Could you check a few things on this drawing? It's one solid part, dimensions in mm from its lowest x, y, z. A direction names the side the tool comes from. Give positions to 0.01 mm unless a question says otherwise; leave off trailing zeros. Write each loop counter-clockwise with the first axis right and the second up, starting at its lowest first coordinate (ties: lowest second). Pieces come first, ordered by that corner, then holes.
1. Suppose I cut it at C-C (x = 24.6). Please give me the cut outline in (y, z), and give its area (3 significant figures).
2. Suppose I cut it at B-B (z = 18). Please give me the cut outline in (x, y), and give its area (4 significant figures).
3. On a 3-axis mill with a long thin cutter (end or side, diameter ignored), from which of +Z, -Z, +X, -X, +Y, -Y can I reach the whole of each face in a straight line? I mean the marked faces 1, 2 and 3. Say none if no direction works.
4. Thinking about a two-plate mould opening in Z: for the marked faces 4, 5 and 6, which applies, pulls with the +Z half, pulls with the -Z half, needs draft (parallel to the pull), parting line crosses it, or undercut?
5. Suppose I cut it at D-D (x = 7). Please give me the cut outline in (y, z), and give its area (3 significant figures).
6. I'm going to push flat-ended pins straight in: pin 1 (0.9 mm diameter, centred on y = 19, z = 1.5, fed in from +X); pin 2 (0.9 mm diameter, centred on y = 17, z = 22.5, fed in from -X); pin 3 (3 mm diameter, centred on x = 23, z = 15.5, fed in from -Y). Where does each tip first touch, or does it pass through?
7. If I drill on probe 1 along Y at (x, z) = (10.8, 21.9); probe 2 along Z at (x, y) = (17.7, 66.85); probe 3 along X at (y, z) = (4, 1.65), over which ranges is the centre line in solid material (lowest first)?
8. Suppose I cut it at A-A (y = 4). Please give me the cut outline in (x, z).
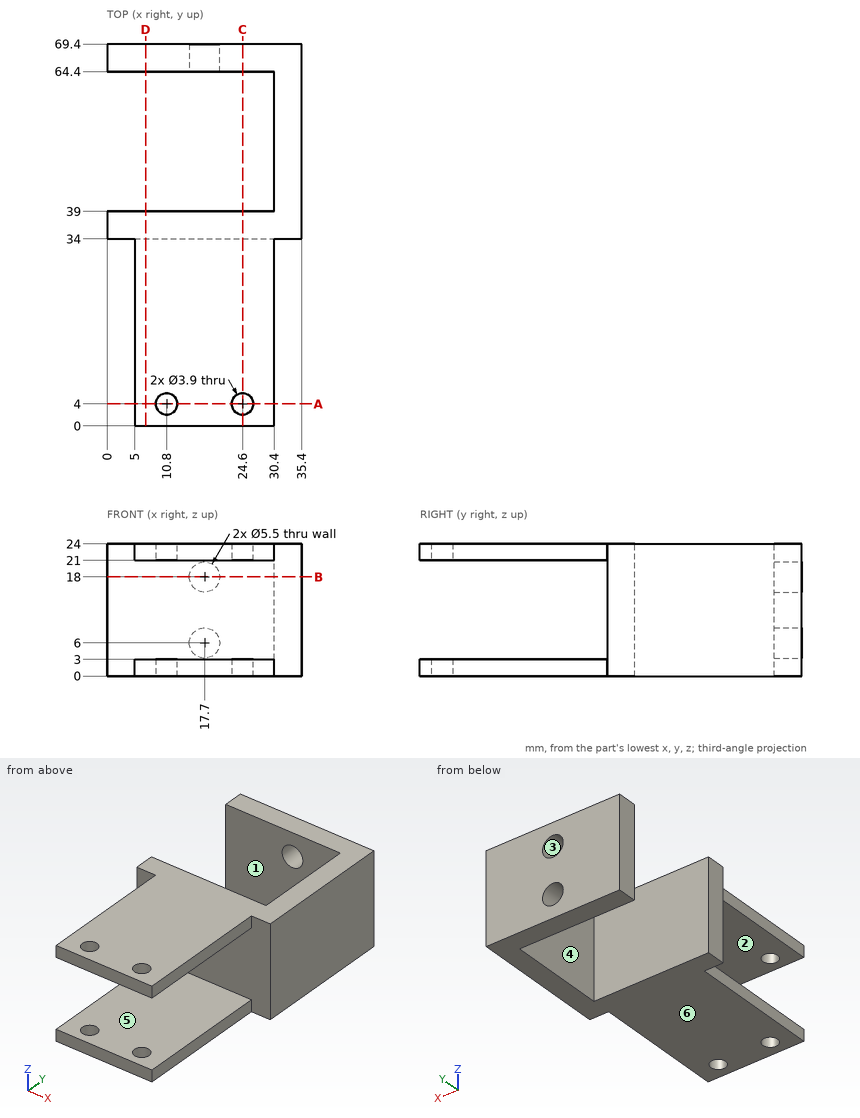
Checks:
1. outline: (0, 0) - (2.05, 0) - (2.05, 3) - (0, 3) - close; (0, 21) - (2.05, 21) - (2.05, 24) - (0, 24) - close; (5.95, 0) - (39, 0) - (39, 24) - (5.95, 24) - (5.95, 21) - (34, 21) - (34, 3) - (5.95, 3) - close; (64.4, 0) - (69.4, 0) - (69.4, 24) - (64.4, 24) - close
1. area: 421 mm2
2. outline: (0, 34) - (35.4, 34) - (35.4, 69.4) - (20.45, 69.4) - (20.45, 64.4) - (30.4, 64.4) - (30.4, 39) - (0, 39) - close; (0, 64.4) - (14.95, 64.4) - (14.95, 69.4) - (0, 69.4) - close
2. area: 453.5 mm2
3. face 1: +Z, -Z, -X
3. face 2: +X, -X, -Y
3. face 3: +Y
4. face 4: needs draft
4. face 5: undercut
4. face 6: pulls with the -Z half
5. outline: (0, 0) - (39, 0) - (39, 24) - (0, 24) - (0, 21) - (34, 21) - (34, 3) - (0, 3) - close; (64.4, 0) - (69.4, 0) - (69.4, 24) - (64.4, 24) - close
5. area: 444 mm2
6. pin 1: stops at x = 30.4
6. pin 2: stops at x = 5
6. pin 3: stops at y = 34
7. probe 1: y = 0 to 2.05, 5.95 to 39, 64.4 to 69.4
7. probe 2: z = 0 to 3.25, 8.75 to 15.25, 20.75 to 24
7. probe 3: x = 5 to 8.85, 12.75 to 22.65, 26.55 to 30.4
8. outline: (5, 0) - (8.85, 0) - (8.85, 3) - (5, 3) - close; (5, 21) - (8.85, 21) - (8.85, 24) - (5, 24) - close; (12.75, 0) - (22.65, 0) - (22.65, 3) - (12.75, 3) - close; (12.75, 21) - (22.65, 21) - (22.65, 24) - (12.75, 24) - close; (26.55, 0) - (30.4, 0) - (30.4, 3) - (26.55, 3) - close; (26.55, 21) - (30.4, 21) - (30.4, 24) - (26.55, 24) - close
